from build123d import *

# Parameters (mm, degrees)
SKETCH2_R               = 18
SKETCH2_W               = 7.5
SKETCH2_H               = 7.5
BOSS_EXTRUDE1_DEPTH     = 1.8
BOSS_EXTRUDE10_START    = 1.8
SKETCH18_W              = 7.7
SKETCH18_H              = 7.7
BOSS_EXTRUDE10_DEPTH    = 1.8
BOSS_EXTRUDE2_START     = -1.8
SKETCH3_R               = 35
SKETCH3_R_2             = 18
BOSS_EXTRUDE2_DEPTH     = 1.8
SKETCH4_R               = 2.9
BOSS_EXTRUDE3_DEPTH     = 3
CUT_EXTRUDE1_DEPTH      = 50.588305073
CUT_EXTRUDE1_DEPTH_BACK = 50.588305073
SKETCH7_R               = 59.131365533
FILLET1_R               = 6


with BuildPart() as part:
    # Sketch2 → Boss-Extrude1 (new body)
    with BuildSketch(Plane.XY.offset(10)):
        Circle(SKETCH2_R)
        with BuildLine():
            Line((-8.15, -8.35), (-8.15, -14.91903147))
            ThreePointArc((-8.15, -14.91903147), (-11.939670478, -12.101415986), (-14.808021475, -8.35))
            Line((-14.808021475, -8.35), (-8.15, -8.35))
        make_face(mode=Mode.SUBTRACT)
        with BuildLine():
            Line((-8.15, -7.85), (-15.079041747, -7.85))
            ThreePointArc((-15.079041747, -7.85), (-16.470304718, -4.210589327), (-16.996396677, -0.35))
            Line((-16.996396677, -0.35), (-8.15, -0.35))
            Line((-8.15, -0.35), (-8.15, -7.85))
        make_face(mode=Mode.SUBTRACT)
        with BuildLine():
            Line((-8.15, 0.15), (-16.999338222, 0.15))
            ThreePointArc((-16.999338222, 0.15), (-16.521617742, 4.00451585), (-15.181485435, 7.65))
            Line((-15.181485435, 7.65), (-8.15, 7.65))
            Line((-8.15, 7.65), (-8.15, 0.15))
        make_face(mode=Mode.SUBTRACT)
        with BuildLine():
            Line((-8.15, 8.15), (-14.91903147, 8.15))
            ThreePointArc((-14.91903147, 8.15), (-12.02081528, 12.02081528), (-8.15, 14.91903147))
            Line((-8.15, 14.91903147), (-8.15, 8.15))
        make_face(mode=Mode.SUBTRACT)
        with BuildLine():
            Line((-7.65, 8.15), (-7.65, 15.181485435))
            ThreePointArc((-7.65, 15.181485435), (-4.00451585, 16.521617742), (-0.15, 16.999338222))
            Line((-0.15, 16.999338222), (-0.15, 8.15))
            Line((-0.15, 8.15), (-7.65, 8.15))
        make_face(mode=Mode.SUBTRACT)
        with BuildLine():
            Line((0.35, 8.15), (0.35, 16.996396677))
            ThreePointArc((0.35, 16.996396677), (4.210589327, 16.470304718), (7.85, 15.079041747))
            Line((7.85, 15.079041747), (7.85, 8.15))
            Line((7.85, 8.15), (0.35, 8.15))
        make_face(mode=Mode.SUBTRACT)
        with BuildLine():
            Line((8.35, 8.15), (8.35, 14.808021475))
            ThreePointArc((8.35, 14.808021475), (12.101415986, 11.939670478), (14.91903147, 8.15))
            Line((14.91903147, 8.15), (8.35, 8.15))
        make_face(mode=Mode.SUBTRACT)
        with BuildLine():
            Line((8.35, 7.65), (15.181485435, 7.65))
            ThreePointArc((15.181485435, 7.65), (16.521617742, 4.00451585), (16.999338222, 0.15))
            Line((16.999338222, 0.15), (8.35, 0.15))
            Line((8.35, 0.15), (8.35, 7.65))
        make_face(mode=Mode.SUBTRACT)
        with BuildLine():
            Line((8.35, -0.35), (16.996396677, -0.35))
            ThreePointArc((16.996396677, -0.35), (16.470304718, -4.210589327), (15.079041747, -7.85))
            Line((15.079041747, -7.85), (8.35, -7.85))
            Line((8.35, -7.85), (8.35, -0.35))
        make_face(mode=Mode.SUBTRACT)
        with BuildLine():
            Line((8.35, -8.35), (14.808021475, -8.35))
            ThreePointArc((14.808021475, -8.35), (12.02081528, -12.02081528), (8.35, -14.808021475))
            Line((8.35, -14.808021475), (8.35, -8.35))
        make_face(mode=Mode.SUBTRACT)
        with BuildLine():
            Line((7.85, -8.35), (7.85, -15.079041747))
            ThreePointArc((7.85, -15.079041747), (4.210589327, -16.470304718), (0.35, -16.996396677))
            Line((0.35, -16.996396677), (0.35, -8.35))
            Line((0.35, -8.35), (7.85, -8.35))
        make_face(mode=Mode.SUBTRACT)
        with BuildLine():
            Line((-0.15, -8.35), (-0.15, -16.999338222))
            ThreePointArc((-0.15, -16.999338222), (-4.00451585, -16.521617742), (-7.65, -15.181485435))
            Line((-7.65, -15.181485435), (-7.65, -8.35))
            Line((-7.65, -8.35), (-0.15, -8.35))
        make_face(mode=Mode.SUBTRACT)
        with Locations((-3.9, -4.1)):
            Rectangle(SKETCH2_W, SKETCH2_H, mode=Mode.SUBTRACT)
        with Locations((4.1, -4.1)):
            Rectangle(SKETCH2_W, SKETCH2_H, mode=Mode.SUBTRACT)
        with Locations((-3.9, 3.9)):
            Rectangle(SKETCH2_W, SKETCH2_H, mode=Mode.SUBTRACT)
        with Locations((4.1, 3.9)):
            Rectangle(SKETCH2_W, SKETCH2_H, mode=Mode.SUBTRACT)
    extrude(amount=-BOSS_EXTRUDE1_DEPTH)

    # Sketch18 → Boss-Extrude10 (add)
    with BuildSketch(Plane.XY.offset(8.2).offset(BOSS_EXTRUDE10_START)):
        with BuildLine():
            ThreePointArc((7.85, 15.079041747), (4.11362184, 16.494790552), (0.15, 16.999338222))
            Line((0.15, 16.999338222), (0.15, 8.15))
            Line((0.15, 8.15), (7.85, 8.15))
            Line((7.85, 8.15), (7.85, 15.079041747))
        make_face()
        with BuildLine():
            Line((8.15, 0.15), (16.999338222, 0.15))
            ThreePointArc((16.999338222, 0.15), (16.494790552, 4.11362184), (15.079041747, 7.85))
            Line((15.079041747, 7.85), (8.15, 7.85))
            Line((8.15, 7.85), (8.15, 0.15))
        make_face()
        with Locations((-4, 4)):
            Rectangle(SKETCH18_W, SKETCH18_H)
        with Locations((4, -4)):
            Rectangle(SKETCH18_W, SKETCH18_H)
        with BuildLine():
            Line((8.15, -8.15), (8.15, -14.91903147))
            ThreePointArc((8.15, -14.91903147), (12.02081528, -12.02081528), (14.91903147, -8.15))
            Line((14.91903147, -8.15), (8.15, -8.15))
        make_face()
        with BuildLine():
            Line((-7.85, -8.15), (-7.85, -15.079041747))
            ThreePointArc((-7.85, -15.079041747), (-4.11362184, -16.494790552), (-0.15, -16.999338222))
            Line((-0.15, -16.999338222), (-0.15, -8.15))
            Line((-0.15, -8.15), (-7.85, -8.15))
        make_face()
        with BuildLine():
            ThreePointArc((-16.999338222, -0.15), (-16.494790552, -4.11362184), (-15.079041747, -7.85))
            Line((-15.079041747, -7.85), (-8.15, -7.85))
            Line((-8.15, -7.85), (-8.15, -0.15))
            Line((-8.15, -0.15), (-16.999338222, -0.15))
        make_face()
        with BuildLine():
            ThreePointArc((-8.15, 14.91903147), (-12.02081528, 12.02081528), (-14.91903147, 8.15))
            Line((-14.91903147, 8.15), (-8.15, 8.15))
            Line((-8.15, 8.15), (-8.15, 14.91903147))
        make_face()
    extrude(amount=-BOSS_EXTRUDE10_DEPTH)

    # Sketch3 → Boss-Extrude2 (add)
    with BuildSketch(Plane(origin=(0, 0, 8.2), x_dir=(-1, 0, 0), z_dir=(0, 0, -1)).offset(BOSS_EXTRUDE2_START)):
        Circle(SKETCH3_R)
        Circle(SKETCH3_R_2, mode=Mode.SUBTRACT)
    extrude(amount=BOSS_EXTRUDE2_DEPTH)

    # Sketch4 → Boss-Extrude3 (add)
    with BuildSketch(Plane(origin=(0, 0, 8.2), x_dir=(-1, 0, 0), z_dir=(0, 0, -1))):
        with Locations((0, 29)):
            Circle(SKETCH4_R)
        with Locations((25.11473671, -14.5)):
            Circle(SKETCH4_R)
        with Locations((-25.11473671, -14.5)):
            Circle(SKETCH4_R)
    extrude(amount=-BOSS_EXTRUDE3_DEPTH)

    # Sketch7 → Cut-Extrude1 (cut, two sides: drawn at the far end of the back side and taken through both)
    with BuildSketch(Plane(origin=(0, 0, 8.2), x_dir=(-1, 0, 0), z_dir=(0, 0, -1)).offset(-CUT_EXTRUDE1_DEPTH_BACK)):
        Circle(SKETCH7_R)
        Polygon((0, 42), (-36.373066959, -21), (36.373066959, -21), align=None, mode=Mode.SUBTRACT)
    extrude(amount=CUT_EXTRUDE1_DEPTH + CUT_EXTRUDE1_DEPTH_BACK, mode=Mode.SUBTRACT)

    # Fillet1
    fillet1_edges = [part.edges().sort_by_distance(p)[0] for p in [
        (4.186533479, 34.748711306, 9.1),
        (32.186533479, -13.748711306, 9.1),
        (28, -21, 9.1),
        (-28, -21, 9.1),
        (-32.186533479, -13.748711306, 9.1),
        (-4.186533479, 34.748711306, 9.1),
    ]]
    fillet(fillet1_edges, radius=FILLET1_R)


solid = part.part
The listing builds one solid part. Answer for the finished solid, in the listing's coordinates (mm). A direction names the side the tool comes from. Give positions to 0.01 mm unless a question says otherwise; leave off trailing zeros. Order: outer loops, then holes, each group sorted by start corner. A loop starts at its lowest first (then second) coordinate and runs counter-clockwise, first axis right, second up. Notation, with made-up numbers: (61, -23) - (71, -23) arc R32 cw to (71, 3) - close; hole circle Ø2 at (7.25, -23.5). An arc over 180 degrees is marked (long way). One line per item, written item: value. Start each with the question number.
1) Find the intervals of material crossed by L1, parallel to Y at x = 6, z = 9.05; L2, parallel to X at y = -12.5, z = 8.35; L3, parallel to X at y = 11, z = 9.65, in increasing order.
2) The mould has two halves that part along Y. Classify faces 1 (the face through (25, -14, 11.2)), 2 (the face through (4, 0.15, 9)), 3 (the face through (-3.67, 34.14, 9.11)): released by +Y, released by -Y, zero draft, split by the parting line, or undercut.
3) A cutting plane is placed at D-D on y = 29. Give the vertices of the cut face in (x, z), then the cut area to 3 significant figures.
4) A cutting plane is placed at C-C on z = 9.15. State how many separate pieces and enclosed holes the cut face has, then the cut area to 3 significant figures.
5) Given pin 1 Ø1.4 at (x, z) = (-2.5, 9) entering from +Y; pin 2 Ø1.4 at (y, z) = (10.5, 9) entering from +X; pin 3 Ø1.4 at (y, z) = (2.5, 8.5) entering from -X, each flat-ended and moving along its own axis, determine where each tip first touches the part or whether it passes through.
6) A cutting plane is placed at B-B on x = 14. Give the vertices of the cut face in (y, z), then the cut area to 3 significant figures.
7) A cutting plane is placed at A-A on y = -5. Give the vertices of the cut face in (x, z), then the cut area to 3 significant figures.
8) A tool of negligible diameter and unlimited length cuts with its end or side. For faces 4 (the face through (7.85, 4, 9)), 5 (the face through (-31.4, -13.9, 9.1)), from which of +Z, -Z, +X, -X, +Y, -Y can it reach the whole face along a straight path? Write none if from no direction.
Answer sheet:
1. L1: y = -21 to -15.91, -8.35 to 0.15, 7.65 to 31.61
1. L2: x = -31.21 to -11.52, -8.15 to 0.35, 7.85 to 31.21
1. L3: x = -17.9 to -7.65, -0.15 to 8.35, 12.96 to 17.9
2. face 1: zero draft
2. face 2: undercut
2. face 3: released by +Y
3. outline: (-7.51, 8.2) - (7.51, 8.2) - (7.51, 10) - (2.9, 10) - (2.9, 11.2) - (-2.9, 11.2) - (-2.9, 10) - (-7.51, 10) - close
3. area: 34.0 mm2
4. separate pieces: 1
4. enclosed holes: 8
4. area: 1,790 mm2
5. pin 1: stops at y = 34.87
5. pin 2: stops at x = 18.59
5. pin 3: stops at x = -23.21
6. outline: (-21, 8.2) - (-7.85, 8.2) - (-7.85, 10) - (-21, 10) - close; (-0.35, 8.2) - (8.15, 8.2) - (8.15, 10) - (-0.35, 10) - close; (9.64, 8.2) - (17.75, 8.2) - (17.75, 10) - (9.64, 10) - close
6. area: 53.6 mm2
7. outline: (-27.14, 8.2) - (-7.65, 8.2) - (-7.65, 10) - (-27.14, 10) - close; (-0.15, 8.2) - (8.35, 8.2) - (8.35, 10) - (-0.15, 10) - close; (16.25, 8.2) - (27.14, 8.2) - (27.14, 10) - (16.25, 10) - close
7. area: 70.0 mm2
8. face 4: +Z, -Z
8. face 5: +Z, -Z, -X
